```python
from build123d import *

# Parameters (mm, degrees)
BOSS_EXTRUDE1_DEPTH       = 15
SKETCH2_W                 = 22
SKETCH2_H                 = 10
CUT_EXTRUDE1_DEPTH        = 10
M2X0_4_TAPPED_HOLE1_D     = 1.6
M2X0_4_TAPPED_HOLE1_DEPTH = 2.75
SKETCH6_W                 = 3
SKETCH6_H                 = 15.5
CUT_EXTRUDE2_DEPTH        = 5
SKETCH7_W                 = 3
SKETCH7_H                 = 10
CUT_EXTRUDE4_DEPTH        = 3
CUT_EXTRUDE5_REACH        = 35.019
SKETCH8_W                 = 5
SKETCH8_H                 = 15


with BuildPart() as part:
    # Sketch1 → Boss-Extrude1 (new body)
    with BuildSketch(Plane(origin=(0, 0, 0), x_dir=(1, 0, 0), z_dir=(0, 1, 0))):
        Polygon((0, -0.563585479), (0, -3.563585479), (25, -3.563585479), (25, 11.936414521), (0, 11.936414521), (0, 8.936414521), (1.5, 8.936414521), (1.5, 10.436414521), (3, 10.436414521), (3, -2.063585479), (1.5, -2.063585479), (1.5, -0.563585479), align=None)
    extrude(amount=BOSS_EXTRUDE1_DEPTH)

    # Sketch2 → Cut-Extrude1 (cut)
    with BuildSketch(Plane(origin=(0, 15, 0), x_dir=(1, 0, 0), z_dir=(0, 1, 0))):
        with Locations((14, 4.186414521)):
            Rectangle(SKETCH2_W, SKETCH2_H)
    extrude(amount=-CUT_EXTRUDE1_DEPTH, mode=Mode.SUBTRACT)

    # M2x0.4 Tapped Hole1
    with Locations(Plane.XY.offset(3.563585479)):
        with Locations((12.5, 10)):
            Hole(M2X0_4_TAPPED_HOLE1_D / 2, depth=M2X0_4_TAPPED_HOLE1_DEPTH)

    # Sketch6 → Cut-Extrude2 (cut)
    with BuildSketch(Plane.XZ):
        with Locations((1.5, -4.186414521)):
            Rectangle(SKETCH6_W, SKETCH6_H)
    extrude(amount=-CUT_EXTRUDE2_DEPTH, mode=Mode.SUBTRACT)

    # Sketch7 → Cut-Extrude4 (cut)
    with BuildSketch(Plane.XY.offset(3.563585479)):
        with Locations((1.5, 10)):
            Rectangle(SKETCH7_W, SKETCH7_H)
    extrude(amount=-CUT_EXTRUDE4_DEPTH, mode=Mode.SUBTRACT)

    # Cut-Extrude5: up to this face of the body (flat: up to its plane)
    cut_extrude5_end = Plane(part.part.faces().sort_by_distance((14, 10, -9.186414521))[0])
    # Sketch8 → Cut-Extrude5 (cut, up to the picked face)
    with BuildSketch(Plane.XY.offset(3.563585479), mode=Mode.PRIVATE) as cut_extrude5_sk1:
        with Locations((5.5, 7.5)):
            Rectangle(SKETCH8_W, SKETCH8_H)
    cut_extrude5_tool1 = split(extrude(cut_extrude5_sk1.sketch, amount=-CUT_EXTRUDE5_REACH, mode=Mode.PRIVATE), bisect_by=cut_extrude5_end, keep=Keep.BOTH, mode=Mode.PRIVATE)
    add(cut_extrude5_tool1.solids().sort_by(Axis((5.5, 7.5, 3.563585), (0, 0, -1)))[0], mode=Mode.SUBTRACT)


solid = part.part
```
The listing builds one solid part. Answer for the finished solid, in the listing's coordinates (mm). A direction names the side the tool comes from. Round coordinates to 2 decimals unless told otherwise and drop trailing zeros. Write each loop counter-clockwise with the first axis right and the second up, starting at its lowest first coordinate (ties: lowest second). Pieces come first, ordered by that corner, then holes. Notation, with made-up numbers: (-17, 19.5) -> (4, 19.5) arc R13 cw to (4, 41.5) -> close; hole circle Ø5 at (10, -37). An arc over 180 degrees is marked (long way). Answer as a JSON object with one key per item and string values. Group by question number.
Q1. Section A-A (y = 13.25) is taken. Write down the section's boundary in (x, z), plus the area to 3 significant figures.
Q2. Section D-D (x = 12.5) is taken. Write down the section's boundary in (y, z).
Q3. Each of these flat-tipped pins is pushed along its axis until it touches: pin 1 Ø6 at (y, z) = (5.5, -5.5) entering from -X; pin 2 Ø4 at (y, z) = (9.5, -2.5) entering from +X; pin 3 Ø1.6 at (x, y) = (2, 12.5) entering from +Z; pin 4 Ø3.5 at (x, z) = (1, -11) entering from -Y. Where does it stop, or does it pass through?
Q4. Which of the six approach directions +Z, -Z, +X, -X, +Y, -Y give full straight-line access (tool end or side, diameter ignored) to faces 1 (the face through (3, 6, -10)), 2 (the face through (2, 10, -10.436)), 3 (the face through (1, 5, -11))?
Q5. Determine the mould class of faces 4 (the face through (16, 10, 0.814)), 5 (the face through (12.604, 10.793, 2.169)), 6 (the face through (25, 4, -4)) for opening direction X: pulls with the +X half, pulls with the -X half, needs draft (parallel to the pull), parting line crosses it, or undercut.
Q6. Section C-C (y = 10) is taken. Write down the section's boundary in (x, z), plus the area to 3 significant figures.
Q7. Straight lines are drawn through the part: line 1 along Z through (x, y) = (22, 8.25); line 2 along Y through (x, z) = (12.5, 1.6); line 3 along X through (y, z) = (3.75, -8.5). For each, find the intervals that lie inside material, in ascending order.
Q8. Section B-B (z = -9.75) is taken. Write down the section's boundary in (x, y).
Check values:
{
 "1": {"outline": "(0, -11.94) -> (25, -11.94) -> (25, -9.19) -> (3, -9.19) -> (3, -10.44) -> (1.5, -10.44) -> (1.5, -8.94) -> (0, -8.94) -> close; (8, 0.81) -> (25, 0.81) -> (25, 3.56) -> (8, 3.56) -> close", "area": "114 mm^2"},
 "2": {"outline": "(0, -11.94) -> (15, -11.94) -> (15, -9.19) -> (5, -9.19) -> (5, 0.81) -> (9.2, 0.81) -> (9.2, 3.56) -> (0, 3.56) -> close; (10.8, 0.81) -> (15, 0.81) -> (15, 3.56) -> (10.8, 3.56) -> close"},
 "3": {"pin 1": "x = 8", "pin 2": "through", "pin 3": "z = -8.94", "pin 4": "y = 5"},
 "4": {"face 1": "+Z, -Y", "face 2": "+Z, +Y, -Y", "face 3": "+Z, -Z, -X, -Y"},
 "5": {"face 4": "needs draft", "face 5": "undercut", "face 6": "pulls with the +X half"},
 "6": {"outline": "(0, -11.94) -> (25, -11.94) -> (25, -9.19) -> (3, -9.19) -> (3, -10.44) -> (1.5, -10.44) -> (1.5, -8.94) -> (0, -8.94) -> close; (8, 0.81) -> (11.7, 0.81) -> (11.7, 3.56) -> (8, 3.56) -> close; (13.3, 0.81) -> (25, 0.81) -> (25, 3.56) -> (13.3, 3.56) -> close", "area": "110 mm^2"},
 "7": {"line 1": "-11.94 to -9.19, 0.81 to 3.56", "line 2": "0 to 9.2, 10.8 to 15", "line 3": "8 to 25"},
 "8": {"outline": "(0, 5) -> (1.5, 5) -> (1.5, 15) -> (0, 15) -> close; (3, 0) -> (25, 0) -> (25, 15) -> (3, 15) -> close"}
}
